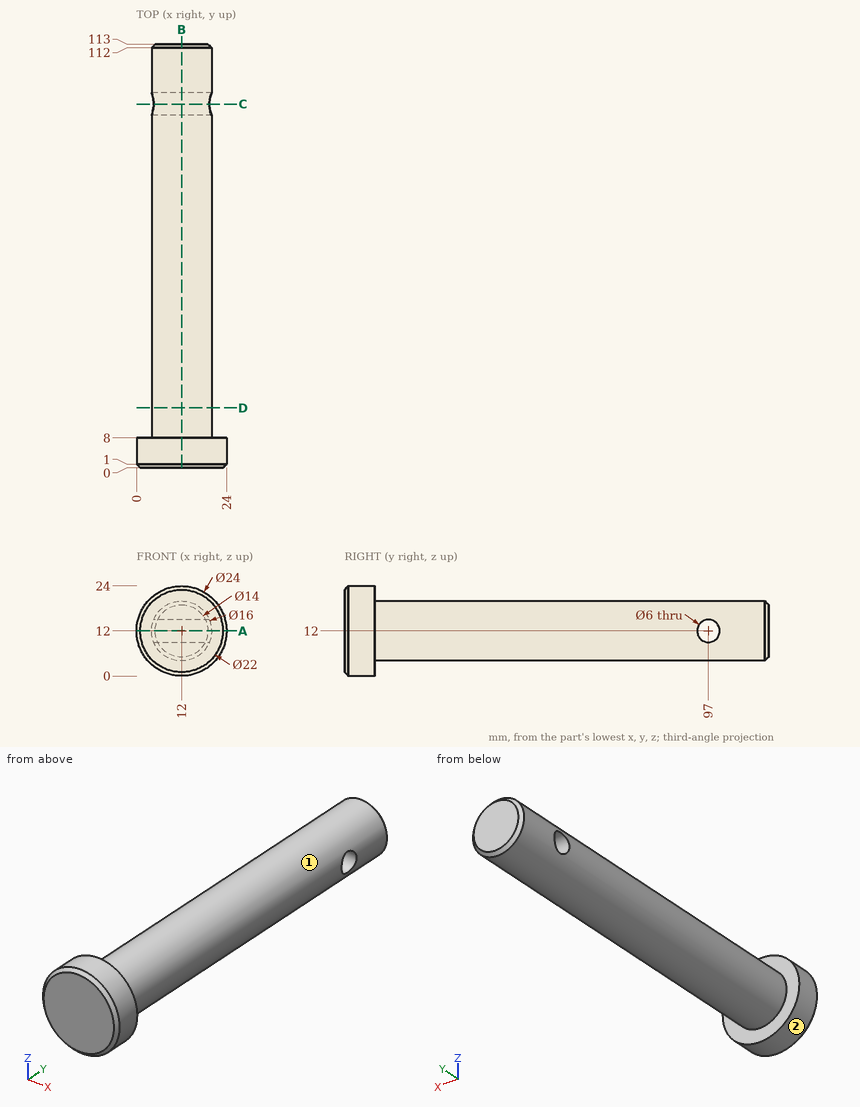
Source: three-view drawing plus pictorial views. Frame: mm from the lowest corner of the part. A direction names the side the tool comes from. Round coordinates to 2 decimals unless told otherwise and drop trailing zeros. Loops run counter-clockwise (first coordinate to the right, second up) from the corner with the lowest first, then second, coordinate; pieces in that order, holes last.
Item 1: Contact query for flat-ended pins moving along their axis: P1, Ø3.5, axis at y = 97, z = 12, coming from the -X side; P2, Ø2, axis at x = 10.5, y = 86.5, coming from the +Z side; P3, Ø2, axis at y = 91, z = 5, coming from the +X side; P4, Ø12, axis at y = 57, z = 19, coming from the -X side. Output: stop coordinate, or through.
Checked values:
P1: passes through
P2: stops at z = 19.98
P3: stops at x = 17.29
P4: stops at x = 4.06
Item 2: Reachability of the marked faces 1 and 2 from +Z, -Z, +X, -X, +Y, -Y: full face, straight path, thin tool, end or side. Return the list, or none.
Checked values:
face 1: +Y
face 2: +Y, -Y
Item 3: Section A-A, the plane z = 12. Output: boundary loops of the cut face in (x, y).
Checked values:
outline: (0, 1) - (1, 0) - (23, 0) - (24, 1) - (24, 8) - (20, 8) - (20, 94) - (4, 94) - (4, 8) - (0, 8) - close; (4, 100) - (20, 100) - (20, 112) - (19, 113) - (5, 113) - (4, 112) - close
Item 4: Section C-C, the plane y = 97. Output: boundary loops of the cut face in (x, z), plus the area to 3 significant figures.
Checked values:
outline: (4.58, 9) arc R8 ccw to (19.42, 9) - close; (4.58, 15) - (19.42, 15) arc R8 ccw to start
area: 107 mm2
Item 5: Section B-B, the plane x = 12. Output: boundary loops of the cut face in (y, z), plus the area to 3 significant figures.
Checked values:
outline: (0, 1) - (1, 0) - (8, 0) - (8, 4) - (112, 4) - (113, 5) - (113, 19) - (112, 20) - (8, 20) - (8, 24) - (1, 24) - (0, 23) - close; hole circle Ø6 at (97, 12)
area: 1,840 mm2
Item 6: Line query: L1, parallel to Y at x = 14.5, z = 12; L2, parallel to Z at x = 12.5, y = 97; L3, parallel to Y at x = 19.75, z = 9.5. Output: solid intervals per line, ascending.
Checked values:
L1: y = 0 to 94, 100 to 113
L2: z = 4.02 to 9, 15 to 19.98
L3: y = 0 to 8
Item 7: Section D-D, the plane y = 16. Output: boundary loops of the cut face in (x, z), plus the area to 3 significant figures.
Checked values:
outline: circle Ø16 at (12, 12)
area: 201 mm2
